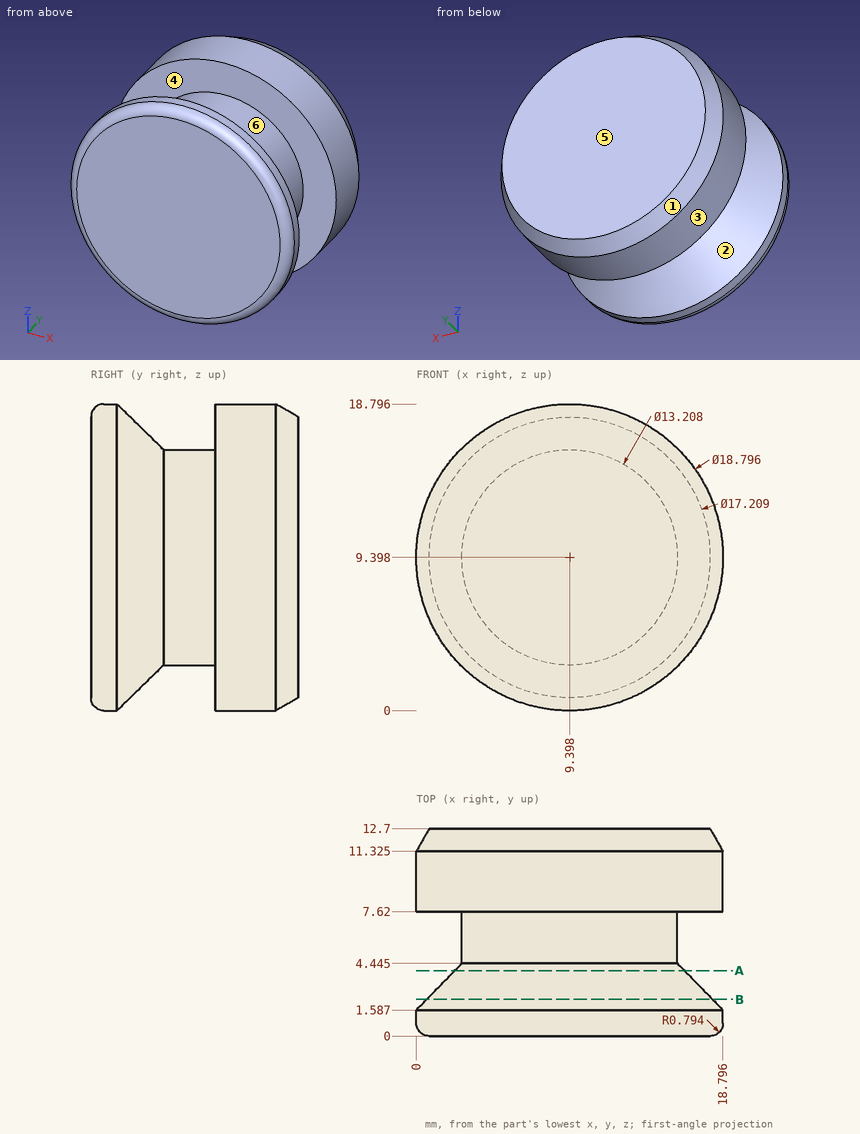
Input: dimensioned drawing with shaded views. Units: mm. Origin: part minimum x, y, z. A direction names the side the tool comes from. Round coordinates to 2 decimals unless told otherwise and drop trailing zeros. Loops run counter-clockwise (first coordinate to the right, second up) from the corner with the lowest first, then second, coordinate; pieces in that order, holes last. Notation, with made-up numbers: (-35, -5) -> (-4, -5) arc R13 cw to (-4, 12) -> close; hole circle Ø7 at (30.5, 19). An arc over 180 degrees is marked (long way). Use one line per item in the form item = value. Start each with the question number.
1) Access query for the marked faces 5 and 6. Directions: +Z, -Z, +X, -X, +Y, -Y. A direction counts if a zero-diameter tool reaches every point of the face in a straight line with its end or side. Return the directions, or none.
2) Line query: L1, parallel to Y at x = 2.75, z = 12.5 (1 decimal); L2, parallel to Y at x = 16.25, z = 4.75; L3, parallel to X at y = 1, z = 13. Output: solid intervals per line, ascending.
3) First-contact query: P1, Ø4, axis at y = 10, z = 13, coming from the +X side; P2, Ø5, axis at x = 13.5, y = 9, coming from the -Z side; P3, Ø2, axis at x = 7, y = 3, coming from the -Z side (1 decimal). Flat tips, straight axial feed; report the tip coordinate or a pass-through.
4) Section A-A on y = 4. Output: boundary loops of the cut face in (x, z).
5) Draft query along Y for the marked faces 1, 2, 3 and 4. Return one class per face: released by +Y, released by -Y, zero draft, split by the parting line, or undercut.
6) Section B-B on y = 2.25. Output: boundary loops of the cut face in (x, z).
Response:
q1.face_5 = +Z, -Z, +X, -X, +Y
q1.face_6 = none
q2.L1 = 0 to 3.7, 7.6 to 12.7
q2.L2 = 0 to 2.73, 7.62 to 12.7
q2.L3 = 0.72 to 18.08
q3.P1 = 18.66
q3.P2 = 0.14
q3.P3 = 0.7
q4.outline = circle Ø14.08 at (9.4, 9.4)
q5.face_1 = released by +Y
q5.face_2 = undercut
q5.face_3 = zero draft
q5.face_4 = undercut
q6.outline = circle Ø17.5 at (9.4, 9.4)
